from build123d import *

# Parameters (mm, degrees)
SQUARE_TUBE_CONFIGURED_20_X_20_X_2_1_DEPTH = 1220
CUT_EXTRUDE_1_REACH                        = 1222.32
SKETCH_2_R                                 = 3.75
SKETCH_3_W                                 = 3
SKETCH_3_H                                 = 20
SKETCH_3_W_2                               = 2.5
CUT_EXTRUDE_2_DEPTH                        = 1221.320142422


with BuildPart() as part:
    # Sketch1 → Square tube - configured 20 X 20 X 2_1 (new body)
    with BuildSketch(Plane(origin=(0, 0, 0), x_dir=(-1, 0, 0), z_dir=(0, 1, 0))):
        with BuildLine():
            Line((-9.5, -12.5), (9.5, -12.5))
            ThreePointArc((9.5, -12.5), (11.621320344, -11.621320344), (12.5, -9.5))
            Line((12.5, -9.5), (12.5, 9.5))
            ThreePointArc((12.5, 9.5), (11.621320344, 11.621320344), (9.5, 12.5))
            Line((9.5, 12.5), (-9.5, 12.5))
            ThreePointArc((-9.5, 12.5), (-11.621320344, 11.621320344), (-12.5, 9.5))
            Line((-12.5, 9.5), (-12.5, -9.5))
            ThreePointArc((-12.5, -9.5), (-11.621320344, -11.621320344), (-9.5, -12.5))
        make_face()
        with BuildLine():
            Line((-9.5, -11), (9.5, -11))
            ThreePointArc((9.5, -11), (10.560660172, -10.560660172), (11, -9.5))
            Line((11, -9.5), (11, 9.5))
            ThreePointArc((11, 9.5), (10.560660172, 10.560660172), (9.5, 11))
            Line((9.5, 11), (-9.5, 11))
            ThreePointArc((-9.5, 11), (-10.560660172, 10.560660172), (-11, 9.5))
            Line((-11, 9.5), (-11, -9.5))
            ThreePointArc((-11, -9.5), (-10.560660172, -10.560660172), (-9.5, -11))
        make_face(mode=Mode.SUBTRACT)
    extrude(amount=SQUARE_TUBE_CONFIGURED_20_X_20_X_2_1_DEPTH)

    # Sketch 2 → Cut-Extrude 1 (cut, up to next)
    with BuildSketch(Plane.ZY.offset(12.5), mode=Mode.PRIVATE) as cut_extrude_1_sk1:
        with Locations((0, 17)):
            Circle(SKETCH_2_R)
    cut_extrude_1_tool1 = extrude(cut_extrude_1_sk1.sketch, amount=-CUT_EXTRUDE_1_REACH, mode=Mode.PRIVATE) & part.part
    # Sketch 2 → Cut-Extrude 1 (cut, up to next)
    with BuildSketch(Plane.ZY.offset(12.5), mode=Mode.PRIVATE) as cut_extrude_1_sk2:
        with Locations((0, 47)):
            Circle(SKETCH_2_R)
    cut_extrude_1_tool2 = extrude(cut_extrude_1_sk2.sketch, amount=-CUT_EXTRUDE_1_REACH, mode=Mode.PRIVATE) & part.part
    cut_extrude_1_1 = cut_extrude_1_tool1.solids().sort_by_distance((-12.5, 17, 0))[0]
    add(cut_extrude_1_1, mode=Mode.SUBTRACT)
    cut_extrude_1_2 = cut_extrude_1_tool2.solids().sort_by_distance((-12.5, 47, 0))[0]
    add(cut_extrude_1_2, mode=Mode.SUBTRACT)
    cut_extrude_1 = cut_extrude_1_1 + cut_extrude_1_2  # Cut-Extrude 1 as one shape, for the pattern or mirror that repeats it

    # Mirror 1: Cut-Extrude 1 across plane
    add(cut_extrude_1.mirror(Plane.ZX.offset(610)), mode=Mode.SUBTRACT)

    # Sketch 3 → Cut-Extrude 2 (cut, through all)
    with BuildSketch(Plane.XY.offset(12.5)):
        with Locations((0, 888.220627209)):
            Rectangle(SKETCH_3_W, SKETCH_3_H)
        with Locations((0, 839.220627209)):
            Rectangle(SKETCH_3_W_2, SKETCH_3_H)
        with Locations((0.25, 689.264040992)):
            Rectangle(SKETCH_3_W, SKETCH_3_H)
        with Locations((0.25, 640.264040992)):
            Rectangle(SKETCH_3_W_2, SKETCH_3_H)
        with Locations((0.5, 490.307454775)):
            Rectangle(SKETCH_3_W, SKETCH_3_H)
        with Locations((0.5, 441.307454775)):
            Rectangle(SKETCH_3_W_2, SKETCH_3_H)
    extrude(amount=-CUT_EXTRUDE_2_DEPTH, mode=Mode.SUBTRACT)


solid = part.part
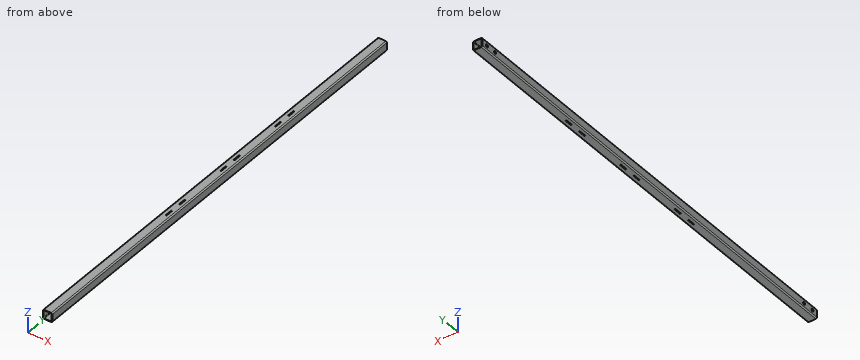
The listing builds one solid part. Answer for the finished solid, in the listing's coordinates (mm). Give positions to 0.01 mm unless a question says otherwise; leave off trailing zeros. Write each loop counter-clockwise with the first axis right and the second up, starting at its lowest first coordinate (ties: lowest second). Pieces come first, ordered by that corner, then holes. Notation, with made-up numbers: (13, -5.5) -> (23, -5.5) arc R25 cw to (23, 15.5) -> close; hole circle Ø5 at (80.25, 83). An arc over 180 degrees is marked (long way). Use a Markdown table: item, result.
(1) Flat-ended cylindrical pins translate along their axes: P1, Ø1, axis at y = 235.5, z = -10, coming from the +X side; P2, Ø0.8, axis at y = 441.5, z = 11.5, coming from the -X side; P3, Ø1.2, axis at y = 688, z = -11.5, coming from the -X side; P4, Ø0.8, axis at y = 442, z = -12, coming from the +X side. Find the tip coordinate at first contact, or state that the pin passes through.
Return value:
| item | result |
|---|---|
| P1 | x = 12.5 |
| P2 | x = -12.04 |
| P3 | x = -12.15 |
| P4 | x = 11.64 |
(2) Section B-B, the plane x = -5.5 is taken. Determine the outline of the cut face in (y, z).
Return value:
| item | result |
|---|---|
| outline | (0, -12.5) -> (1220, -12.5) -> (1220, -11) -> (0, -11) -> close; (0, 11) -> (1220, 11) -> (1220, 12.5) -> (0, 12.5) -> close |
(3) Section C-C, the plane z = 0 is taken. Determine the outline of the cut face in (x, y), then the cut area to 4 significant figures.
Return value:
| item | result |
|---|---|
| outline | (-12.5, 0) -> (-11, 0) -> (-11, 13.25) -> (-12.5, 13.25) -> close; (-12.5, 20.75) -> (-11, 20.75) -> (-11, 43.25) -> (-12.5, 43.25) -> close; (-12.5, 50.75) -> (-11, 50.75) -> (-11, 1169.25) -> (-12.5, 1169.25) -> close; (-12.5, 1176.75) -> (-11, 1176.75) -> (-11, 1199.25) -> (-12.5, 1199.25) -> close; (-12.5, 1206.75) -> (-11, 1206.75) -> (-11, 1220) -> (-12.5, 1220) -> close; (11, 0) -> (12.5, 0) -> (12.5, 1220) -> (11, 1220) -> close |
| area | 3,615 mm2 |
(4) Section A-A, the plane y = 592 is taken. Determine the outline of the cut face in (x, z), then the cut area to 3 significant figures.
Return value:
| item | result |
|---|---|
| outline | (-12.5, -9.5) arc R3 ccw to (-9.5, -12.5) -> (9.5, -12.5) arc R3 ccw to (12.5, -9.5) -> (12.5, 9.5) arc R3 ccw to (9.5, 12.5) -> (-9.5, 12.5) arc R3 ccw to (-12.5, 9.5) -> close; hole (-11, -9.5) arc R1.5 ccw to (-9.5, -11) -> (9.5, -11) arc R1.5 ccw to (11, -9.5) -> (11, 9.5) arc R1.5 ccw to (9.5, 11) -> (-9.5, 11) arc R1.5 ccw to (-11, 9.5) -> close |
| area | 135 mm2 |
(5) Find the intervals of material crossed by probe 1 along Y at (x, z) = (-12.1, 0); probe 2 along Z at (x, y) = (-0.75, 1071.5); probe 3 along Z at (x, y) = (-12, 1203), in increasing order. Write a range as from..to.
Return value:
| item | result |
|---|---|
| probe 1 | 0..13.25, 20.75..43.25, 50.75..1169.25, 1176.75..1199.25, 1206.75..1220 |
| probe 2 | -12.5..-11, 11..12.5 |
| probe 3 | -11.16..-3.75, 3.75..11.16 |
